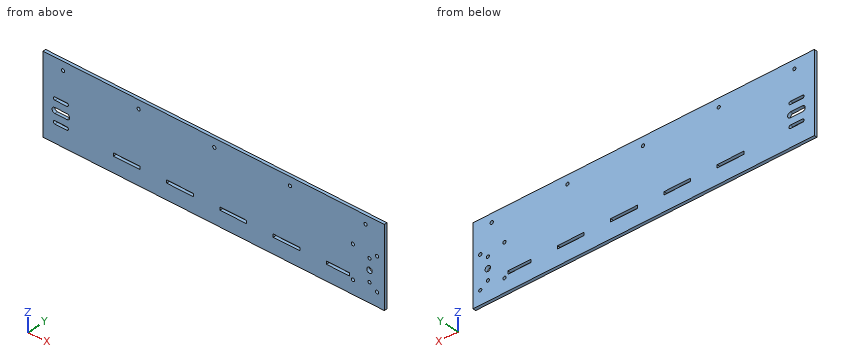
```python
from build123d import *

# Parameters (mm, degrees)
SKETCH1_R           = 2.65
SKETCH1_R_2         = 2.55
SKETCH1_R_3         = 4.5
SKETCH1_W           = 38
SKETCH1_H           = 5
SKETCH1_W_2         = 44
BOSS_EXTRUDE1_DEPTH = 5


with BuildPart() as part:
    # Sketch1 → Boss-Extrude1 (new body)
    with BuildSketch(Plane(origin=(0, 0, 0), x_dir=(1, 0, 0), z_dir=(0, 1, 0))):
        Polygon((0, 0), (0, 40), (0, 65), (-564, 65), (-564, -65), (-524.5, -65), (0, -65), align=None)
        with Locations(Location((-12, 42.5, 0), (0, 0, 270))):
            Circle(SKETCH1_R, mode=Mode.SUBTRACT)
        with Locations(Location((-24.5, 33.5, 0), (0, 0, 270))):
            Circle(SKETCH1_R_2, mode=Mode.SUBTRACT)
        with Locations(Location((-24.5, -2.5, 0), (0, 0, 270))):
            Circle(SKETCH1_R_2, mode=Mode.SUBTRACT)
        with Locations(Location((-24.5, 15.5, 0), (0, 0, 270))):
            Circle(SKETCH1_R_3, mode=Mode.SUBTRACT)
        with Locations(Location((-12, -11.5, 0), (0, 0, 270))):
            Circle(SKETCH1_R, mode=Mode.SUBTRACT)
        with Locations(Location((-531, -51, 0), (0, 0, 270))):
            Circle(SKETCH1_R, mode=Mode.SUBTRACT)
        with Locations(Location((-406, -51, 0), (0, 0, 270))):
            Circle(SKETCH1_R, mode=Mode.SUBTRACT)
        with Locations(Location((-281, -51, 0), (0, 0, 270))):
            Circle(SKETCH1_R, mode=Mode.SUBTRACT)
        with Locations(Location((-156, -51, 0), (0, 0, 270))):
            Circle(SKETCH1_R, mode=Mode.SUBTRACT)
        with Locations(Location((-52, -11.5, 0), (0, 0, 270))):
            Circle(SKETCH1_R, mode=Mode.SUBTRACT)
        with Locations(Location((-52, 42.5, 0), (0, 0, 270))):
            Circle(SKETCH1_R, mode=Mode.SUBTRACT)
        with Locations(Location((-31, -51, 0), (0, 0, 270))):
            Circle(SKETCH1_R, mode=Mode.SUBTRACT)
        with Locations((-76.559496053, 37)):
            Rectangle(SKETCH1_W, SKETCH1_H, mode=Mode.SUBTRACT)
        with BuildLine():
            Line((-544.5, 36.05), (-524.5, 36.05))
            ThreePointArc((-524.5, 36.05), (-521.95, 33.5), (-524.5, 30.95))
            Line((-524.5, 30.95), (-544.5, 30.95))
            ThreePointArc((-544.5, 30.95), (-547.05, 33.5), (-544.5, 36.05))
        make_face(mode=Mode.SUBTRACT)
        with BuildLine():
            Line((-524.5, 0.05), (-544.5, 0.05))
            ThreePointArc((-544.5, 0.05), (-547.05, -2.5), (-544.5, -5.05))
            Line((-544.5, -5.05), (-524.5, -5.05))
            ThreePointArc((-524.5, -5.05), (-521.95, -2.5), (-524.5, 0.05))
        make_face(mode=Mode.SUBTRACT)
        with BuildLine():
            Line((-544.5, 20), (-524.5, 20))
            ThreePointArc((-524.5, 20), (-520, 15.5), (-524.5, 11))
            Line((-524.5, 11), (-544.5, 11))
            ThreePointArc((-544.5, 11), (-549, 15.5), (-544.5, 20))
        make_face(mode=Mode.SUBTRACT)
        with Locations((-161.559496053, 37)):
            Rectangle(SKETCH1_W_2, SKETCH1_H, mode=Mode.SUBTRACT)
        with Locations((-249.559496053, 37)):
            Rectangle(SKETCH1_W_2, SKETCH1_H, mode=Mode.SUBTRACT)
        with Locations((-337.559496053, 37)):
            Rectangle(SKETCH1_W_2, SKETCH1_H, mode=Mode.SUBTRACT)
        with Locations((-425.559496053, 37)):
            Rectangle(SKETCH1_W_2, SKETCH1_H, mode=Mode.SUBTRACT)
    extrude(amount=BOSS_EXTRUDE1_DEPTH)


solid = part.part
```
Geometry check sheet. Reference: the model listing, model coordinates, mm. Give positions to 0.01 mm unless a question says otherwise; leave off trailing zeros. Write each loop counter-clockwise with the first axis right and the second up, starting at its lowest first coordinate (ties: lowest second). Pieces come first, ordered by that corner, then holes. Notation, with made-up numbers: (89, 11.25) -> (114, 11.25) arc R21 ccw to (114, 36.25) -> close; hole circle Ø4 at (21, 81.5). An arc over 180 degrees is marked (long way). One line per question, with ' | ' between items.
Item 1: Sectioned sample at B-B, the plane y = 4.1. State how many separate pieces and enclosed holes the cut face has, plus the area to 3 significant figures.
Determined:
separate pieces: 1 | enclosed holes: 20 | area: 71,500 mm^2
Item 2: Scan lines: line 1 along Z through (x, y) = (-156, 1.45); line 2 along X through (y, z) = (4.6, -37); line 3 along Z through (x, y) = (-281, 2.75). Record each from-to range of solid material in increasing order.
Determined:
line 1: -65 to -39.5, -34.5 to 48.35, 53.65 to 65 | line 2: -564 to -447.56, -403.56 to -359.56, -315.56 to -271.56, -227.56 to -183.56, -139.56 to -95.56, -57.56 to 0 | line 3: -65 to 48.35, 53.65 to 65
Item 3: Sectioned sample at A-A, the plane x = -332. Record the boundary of the cut face in (y, z), plus the area to 3 significant figures.
Determined:
outline: (0, -65) -> (5, -65) -> (5, -39.5) -> (0, -39.5) -> close; (0, -34.5) -> (5, -34.5) -> (5, 65) -> (0, 65) -> close | area: 625 mm^2
